from build123d import *

# Parameters (mm, degrees)
F0_R     = 12.7
F1_DEPTH = 63.5
F3_DEPTH = 25.4
F4_R     = 3.175
F5_DEPTH = 19.051


with BuildPart() as f1:
    # F0 (on Right) → F1 (new body, symmetric)
    with BuildSketch(Plane.YZ):
        Circle(F0_R)
    extrude(amount=F1_DEPTH, both=True)

    # F2 (on face) → F3 (cut)
    with BuildSketch(Plane.YZ.offset(63.5)):
        with BuildLine():
            Line((10.998523, -6.35), (-10.998523, -6.35))
            ThreePointArc((-10.998523, -6.35), (0, -12.7), (10.998523, -6.35))
        make_face()
        with BuildLine():
            ThreePointArc((10.998523, 6.35), (0, 12.7), (-10.998523, 6.35))
            Line((-10.998523, 6.35), (10.998523, 6.35))
        make_face()
    extrude(amount=-F3_DEPTH, mode=Mode.SUBTRACT)

    # F4 (on face) → F5 (cut, through all)
    with BuildSketch(Plane.XY.offset(6.35)):
        with Locations((57.15, 0)):
            Circle(F4_R)
    extrude(amount=-F5_DEPTH, mode=Mode.SUBTRACT)


solid = f1.part
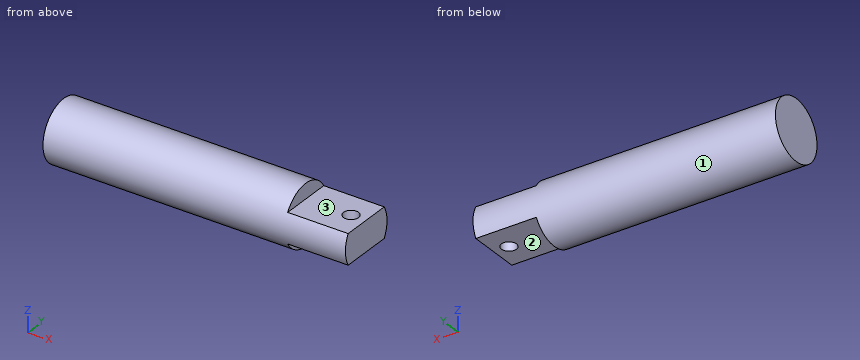
Geometry: final body of the model. Coordinates: model frame, mm. Face numbers are marked on the shaded views. A direction names the side the tool comes from. Give positions to 0.01 mm unless a question says otherwise; leave off trailing zeros. Order: outer loops, then holes, each group sorted by start corner. A loop starts at its lowest first (then second) coordinate and runs counter-clockwise, first axis right, second up. Notation, with made-up numbers: (43.5, -11) -> (101.5, -11) arc R14 ccw to (101.5, -5) -> close; hole circle Ø8 at (89.5, 87.25). An arc over 180 degrees is marked (long way). Answer as a JSON object with one key per item and string values.
Q1. Access query for the marked faces 1, 2 and 3. Directions: +Z, -Z, +X, -X, +Y, -Y. A direction counts if a zero-diameter tool reaches every point of the face in a straight line with its end or side. Return the directions, or none.
Entries:
{"face 1": "+X, -X", "face 2": "-Z, +X, +Y, -Y", "face 3": "+Z, +X, +Y, -Y"}
Q2. Section B-B (x = 57.15). Output: boundary loops of the cut face in (y, z) (3 decimals).
Entries:
{"outline": "(-10.999, -6.35) -> (-3.175, -6.35) -> (-3.175, 6.35) -> (-10.999, 6.35) arc R12.7 ccw to start; (3.175, -6.35) -> (10.999, -6.35) arc R12.7 ccw to (10.999, 6.35) -> (3.175, 6.35) -> close"}
Q3. Section C-C (z = -5). Output: boundary loops of the cut face in (x, y) (3 decimals), plus the area to 3 significant figures.
Entries:
{"outline": "(-63.5, -11.674) -> (63.5, -11.674) -> (63.5, 11.674) -> (-63.5, 11.674) -> close; hole circle Ø6.35 at (57.15, 0)", "area": "2,930 mm^2"}
Q4. Section D-D (y = -9.5). Output: boundary loops of the cut face in (x, z).
Entries:
{"outline": "(-63.5, -8.43) -> (38.1, -8.43) -> (38.1, -6.35) -> (63.5, -6.35) -> (63.5, 6.35) -> (38.1, 6.35) -> (38.1, 8.43) -> (-63.5, 8.43) -> close"}
Q5. Section A-A (y = 0). Output: boundary loops of the cut face in (x, z) (3 decimals).
Entries:
{"outline": "(-63.5, -12.7) -> (38.1, -12.7) -> (38.1, -6.35) -> (53.975, -6.35) -> (53.975, 6.35) -> (38.1, 6.35) -> (38.1, 12.7) -> (-63.5, 12.7) -> close; (60.325, -6.35) -> (63.5, -6.35) -> (63.5, 6.35) -> (60.325, 6.35) -> close"}
Q6. First-contact query: pin 1 (1 mm diameter, centred on x = -27.5, y = 8.5, fed in from +Z); pin 2 (8 mm diameter, centred on x = -23.5, y = 8, fed in from +Z); pin 3 (10 mm diameter, centred on x = -29, z = 8, fed in from -Y); pin 4 (12 mm diameter, centred on x = 33, y = 4, fed in from +Z). Flat tips, straight axial feed; report the tip coordinate or a pass-through.
Entries:
{"pin 1": "stops at z = 9.86", "pin 2": "stops at z = 12.05", "pin 3": "stops at y = -12.34", "pin 4": "stops at z = 12.7"}
Q7. Material intervals for probe 1 along Y at (x, z) = (29, 0); probe 2 along Z at (x, y) = (-20.5, 0.5); probe 3 along X at (y, z) = (2, 6.75), sorted ascending.
Entries:
{"probe 1": "y = -12.7 to 12.7", "probe 2": "z = -12.69 to 12.69", "probe 3": "x = -63.5 to 38.1"}
